Read the model definition and answer for the solid it produces. Units are mm, in the model's axes. A direction names the side the tool comes from. Coordinates: 2 decimals unless noted, no trailing zeros. Order: outer loops, then holes, each group sorted by start corner. A loop starts at its lowest first (then second) coordinate and runs counter-clockwise, first axis right, second up. Notation, with made-up numbers: M 80,1.25 L 101,1.25 A30 cw 101,26.25 Z; hole C -38,2.25 d4. An arc over 180 degrees is marked long. Put each result on its own line as item: value.
from build123d import *

# Parameters (mm, degrees)
SKETCH1_W                                           = 36
SKETCH1_H                                           = 45
BOSS_EXTRUDE1_DEPTH                                 = 5
M2_TAPPED_HOLE1_D                                   = 1.6
M2_TAPPED_HOLE1_DEPTH                               = 5
M2_TAPPED_HOLE1_TIP                                 = 0.480688495
CSK_FOR_M2_COUNTERSUNK_FLAT_HEAD_SCREW1_D           = 2.4
CSK_FOR_M2_COUNTERSUNK_FLAT_HEAD_SCREW1_CSINK_D     = 4.4
CSK_FOR_M2_COUNTERSUNK_FLAT_HEAD_SCREW1_CSINK_ANGLE = 90


with BuildPart() as part:
    # Sketch1 → Boss-Extrude1 (new body)
    with BuildSketch(Plane(origin=(0, 0, 0), x_dir=(0, 0, -1), z_dir=(1, 0, 0))):
        Rectangle(SKETCH1_W, SKETCH1_H)
    extrude(amount=BOSS_EXTRUDE1_DEPTH)

    # M2 Tapped Hole1
    with Locations(Plane(origin=(0, 22.5, 0), x_dir=(1, 0, 0), z_dir=(0, 1, 0))):
        with Locations((2.5, 7.5), (2.5, -7.5)):
            Hole(M2_TAPPED_HOLE1_D / 2, depth=M2_TAPPED_HOLE1_DEPTH)
            with Locations((0, 0, -(M2_TAPPED_HOLE1_DEPTH + M2_TAPPED_HOLE1_TIP / 2))):  # 118° drill point
                Cone(0, M2_TAPPED_HOLE1_D / 2, M2_TAPPED_HOLE1_TIP, mode=Mode.SUBTRACT)

    # CSK for M2 Countersunk Flat Head Screw1 (through all)
    with Locations(Plane(origin=(5, 0, 0), x_dir=(0, 0, -1), z_dir=(1, 0, 0))):
        with Locations((-9, -20), (9, -20)):
            CounterSinkHole(CSK_FOR_M2_COUNTERSUNK_FLAT_HEAD_SCREW1_D / 2, CSK_FOR_M2_COUNTERSUNK_FLAT_HEAD_SCREW1_CSINK_D / 2, counter_sink_angle=CSK_FOR_M2_COUNTERSUNK_FLAT_HEAD_SCREW1_CSINK_ANGLE)


solid = part.part
Q1. Given pin 1 (3 mm diameter, centred on y = -20, z = 9, fed in from +X), flat-ended and moving along its own axis, determine where the tip first touches the part or whether it passes through.
Answers below:
pin 1: stops at x = 4.3
Q2. Consider line 1 along Z through (x, y) = (3, -20); line 2 along Y through (x, z) = (2.8, 9); line 3 along Z through (x, y) = (2.5, 18.95). Determine where each line is inside the solid, lowest interval first.
Answers below:
line 1: z = -18 to -10.2, -7.8 to 7.8, 10.2 to 18
line 2: y = -22.5 to -21.2, -18.8 to 22.5
line 3: z = -18 to -8.3, -6.7 to 6.7, 8.3 to 18
Q3. Find section A-A on z = 9. Write down the section's boundary in (x, y), plus the area to 3 significant figures.
Answers below:
outline: M 0,-22.5 L 5,-22.5 L 5,-22.2 L 4,-21.2 L 0,-21.2 Z; M 0,-18.8 L 4,-18.8 L 5,-17.8 L 5,22.5 L 0,22.5 Z
area: 212 mm^2
Q4. A tool of negligible diameter and unlimited length cuts with its end or side. For faces 1 (the face through (5, 0, 0)), 2 (the face through (3.09, 19.96, 6.96)), from which of +Z, -Z, +X, -X, +Y, -Y can it reach the whole face along a straight path? Write none if from no direction.
Answers below:
face 1: +Z, -Z, +X, +Y, -Y
face 2: +Y
Q5. For a pull along Z with two mould halves and no side action, classify faces 3 (the face through (2, 0, -18)), 4 (the face through (2.604, 19.965, -8.293)), 5 (the face through (1.97, -21.17, 8.74)), 6 (the face through (2, -22.5, 0)) as +Z half, -Z half, draft (parallel to the pull), parting line (faces both ways), or undercut.
Answers below:
face 3: -Z half
face 4: undercut
face 5: undercut
face 6: draft
